For this review, take the finished solid that the model builds, in its own axes (mm). A direction names the side the tool comes from. Give positions to 0.01 mm unless a question says otherwise; leave off trailing zeros. Loops run counter-clockwise (first coordinate to the right, second up) from the corner with the lowest first, then second, coordinate; pieces in that order, holes last.
Autodesk Inventor part; units mm, degrees
ref_plane "YZ Plane" through (0, 0, 0) normal (1, 0, 0) x (0, 1, 0)
ref_plane "XZ Plane" through (0, 0, 0) normal (0, 1, 0) x (-1, 0, 0)
ref_plane "XY Plane" through (0, 0, 0) normal (0, 0, 1) x (1, 0, 0)
sketch "Sketch1" plane through (0, 0, 0) normal (0, 1, 0) x (-1, 0, 0)
  line L0 (10, 20) -> (-10, 20)
  line L1 (-10, 20) -> (-10, -20)
  line L2 (-10, -20) -> (10, -20)
  line L3 (10, -20) -> (10, 20)
  line L4 (21, 0) -> (-27, 0) construction
  line L5 (0, 26) -> (0, -28) construction
  line L6 (9.5, 20) -> (9.5, 27)
  line L7 (-9.5, 27) -> (-9.5, 20)
  line L8 (0.5, 20) -> (0.5, 27)
  line L9 (-0.5, 27) -> (-0.5, 20)
  arc A0 (4, 26.2656) -> (6, 26.2656) centre (5, 24.25) ccw
  line L10 (6, 27) -> (6, 26.2656)
  line L11 (4, 27) -> (4, 26.2656)
  line L12 (9.5, 27) -> (6, 27)
  arc A1 (-6, 26.2656) -> (-4, 26.2656) centre (-5, 24.25) ccw
  line L13 (-6, 27) -> (-6, 26.2656)
  line L14 (-4, 27) -> (-4, 26.2656)
  line L15 (4, 27) -> (-4, 27)
  line L16 (-6, 27) -> (-9.5, 27)
  line L17 (9.5, -20) -> (9.5, -27)
  line L18 (-9.5, -27) -> (-9.5, -20)
  line L19 (0.5, -20) -> (0.5, -27)
  line L20 (-0.5, -27) -> (-0.5, -20)
  arc A2 (6, -26.2656) -> (4, -26.2656) centre (5, -24.25) ccw
  line L21 (6, -27) -> (6, -26.2656)
  line L22 (4, -27) -> (4, -26.2656)
  line L23 (9.5, -27) -> (6, -27)
  line L24 (-6, -27) -> (-6, -26.2656)
  arc A3 (-4, -26.2656) -> (-6, -26.2656) centre (-5, -24.25) ccw
  line L25 (-4, -27) -> (-4, -26.2656)
  line L26 (4, -27) -> (-4, -27)
  line L27 (-6, -27) -> (-9.5, -27)
  arc A4 (-8.75, -5.1588) -> (8.75, -5.1588) centre (0, -10) ccw
  line L28 (8.75, 14.5) -> (-8.75, 14.5)
  line L29 (8.75, 14.5) -> (8.75, -5.1588)
  line L30 (-8.75, 14.5) -> (-8.75, -5.1588)
  circle A5 centre (0, -10) radius 6.5
  circle A6 centre (0, -10) radius 5
  circle A7 centre (0, -10) radius 3
  line L31 (9.5, -20) -> (-9.5, -20)
  line L32 (0.5, -20) -> (0.5, -27)
  line L33 (-0.5, -27) -> (-0.5, -20)
  point P0 (0, 0)
  dimension "d0" = 20
  dimension "d1" = 40
  dimension "d5" = 20
  dimension "d6" = 10
  dimension "d10" = 19
  dimension "d11" = 0.5
  dimension "d12" = 0.5
  dimension "d13" = 1
  dimension "d14" = 4.5
  dimension "d15" = 4.25
  dimension "d16" = 4.5
  dimension "d17" = 2
  dimension "d18" = 1
  dimension "d19" = 7
  dimension "d20" = 10
  dimension "d21" = 5.5
  dimension "d22" = 1.25
  dimension "d23" = 13
  dimension "d24" = 10
  dimension "d25" = 6
extrude "Extrusion1" add sketch "Sketch1" along normal blind 1.8 contours L3 A4 L29 L28 L30 L1 L0 | L0 L8 L15 L11 A0 L10 L12 L6 | L3 L2 A4 | A4 L30 L28 L29 | L0 L9 L15 L8 | L2 L19 L26 L20 | L2 L1 A4 | L0 L7 L16 L13 A1 L14 L15 L9 | L17 L23 L21 A2 L22 L26 L19 L2 | L20 L26 L25 A3 L24 L27 L18 L2 | A5 | A6 | A7
extrude "Extrusion2" add sketch "Sketch1" along normal blind 9 contours L3 A4 L29 L28 L30 L1 L0 | L3 L2 A4 | A4 L30 L28 L29 | L2 L1 A4 | A5 | A6 | A7
extrude "Extrusion3" add sketch "Sketch1" along normal blind 11 contours A4 L30 L28 L29
extrude "Extrusion4" cut sketch "Sketch1" along normal blind 12 contours A5
extrude "Extrusion5" add sketch "Sketch1" along normal blind 12 contours A5
extrude "Extrusion6" add sketch "Sketch1" along normal blind 12.5 contours A6
extrude "Extrusion7" cut sketch "Sketch1" along normal blind 17 contours A7
extrude "Extrusion8" add sketch "Sketch1" along normal blind 17 contours A7
extrude "Extrusion9" add sketch "Sketch1" against normal blind 27.5 contours L3 A4 L29 L28 L30 L1 L0 | L3 L2 A4 | A4 L30 L28 L29 | L2 L1 A4 | A5 | A6 | A7
fillet "Fillet1" radius 1 4 edges at (9.5, 0.9, -27) (-9.5, 0.9, -27) (9.5, 0.9, 27) (-9.5, 0.9, 27)
fillet "Fillet2" radius 1 1 edges at (3, 17, -10)
chamfer "Chamfer1" distance 2 angle 45 4 edges at (10, -27.5, 0) (0, -27.5, 20) (-10, -27.5, 0) (0, -27.5, -20)
properties part number "MG996R"
Item 1: For L1, parallel to X at y = 1.4, z = 24.25; L2, parallel to Z at x = 5, y = 0.8; L3, parallel to Y at x = 2, z = 9, list the stretches that pass through material, from the lowest coordinate up.
Answer:
L1: x = -9.5 to -7.25, -2.75 to 2.75, 7.25 to 9.5
L2: z = -22 to 22
L3: y = -27.5 to 11
Item 2: Take a section at A-A on z = -24.25. Give the boundary of the cut face in (x, y).
Answer:
outline: (-9.5, 0) - (-7.25, 0) - (-7.25, 1.8) - (-9.5, 1.8) - close; (-2.75, 0) - (2.75, 0) - (2.75, 1.8) - (-2.75, 1.8) - close; (7.25, 0) - (9.5, 0) - (9.5, 1.8) - (7.25, 1.8) - close
Item 3: Clearance check with flat-ended pins moving along their axes: pin 1 Ø2 at (x, z) = (-3, 19) entering from +Y; pin 2 Ø3 at (x, y) = (1, -4.5) entering from -Z; pin 3 Ø1.4 at (y, z) = (1, -24.5) entering from +X. State where each tip first meets the part, or that it passes through.
Answer:
pin 1: stops at y = 9
pin 2: stops at z = -20
pin 3: stops at x = 9.5
Item 4: The part is to be moulded in two halves that separate along Z. For faces 5 (the cylindrical face through (-5, 1, 22)), 6 (the cylindrical face through (5, 1, -22)), 7 (the flat face through (-9.5, 1, -23)), 8 (the flat face through (7, 1, -27)), say which applies: released by +Z, released by -Z, zero draft, split by the parting line, or undercut.
Answer:
face 5: undercut
face 6: undercut
face 7: zero draft
face 8: released by -Z
Item 5: Take a section at C-C on y = -8. Give the boundary of the cut face in (x, z).
Answer:
outline: (-10, -20) - (10, -20) - (10, 20) - (-10, 20) - close
Item 6: Tool access review of faces 1 (the cylindrical face through (0, 10, -20)), 2 (the flat face through (0, 9, 15)), 3 (the flat face through (0, 1.8, 24)), 4 (the flat face through (8, 9, -18)): name each direction out of +Z, -Z, +X, -X, +Y, -Y from which nothing blocks a thin tool from reaching the whole face with its end or side.
Answer:
face 1: +Y
face 2: +Z, +Y
face 3: +Z, +X, -X, +Y
face 4: -Z, +X, +Y
Item 7: Take a section at B-B on z = 11. Give the boundary of the cut face in (x, y), and give its area (3 significant figures).
Answer:
outline: (-10, -25.5) - (-8, -27.5) - (8, -27.5) - (10, -25.5) - (10, 9) - (8.75, 9) - (8.75, 11) - (-8.75, 11) - (-8.75, 9) - (-10, 9) - close
area: 761 mm2
